Check sheet for the modelled part. Datum: model origin and axes. Units: mm. Coordinates: 2 decimals unless noted, no trailing zeros. Order: outer loops, then holes, each group sorted by start corner. A loop starts at its lowest first (then second) coordinate and runs counter-clockwise, first axis right, second up.
1. Gauge pin test, flat ends, axial feed: pin 1 Ø8 at (y, z) = (-46.5, 55) entering from +X; pin 2 Ø8 at (x, y) = (58, 35.5) entering from -Z; pin 3 Ø6 at (x, z) = (-19.5, 42.5) entering from +Y. Record the tip position at first contact, or that the pin passes through.
2. Cross-section at B-B (x = -5.5). Enter the section's corners in (y, z).
3. Cross-section at D-D (z = 69). Enter the section's corners in (x, y).
4. Cross-section at C-C (y = 25). Enter the section's corners in (x, z), then the cut area to 3 significant figures.
5. Thickness scan on line 1 (X direction, y = 51, z = 74); line 2 (Y direction, x = -110.5, z = 55); line 3 (Y direction, x = 2, z = 70). Record the ranges inside material, lowest first.
6. Cross-section at A-A (z = 39.5). Enter the section's corners in (x, y), then the cut area to 3 significant figures.
```python
from build123d import *

# Parameters (mm, degrees)
F2_DEPTH = 50.8
F4_DEPTH = 254.001


with BuildPart() as f2:
    # F1 (on offset) → F2 (new body)
    with BuildSketch(Plane.XY.offset(25.4)):
        Polygon((0, 127), (-152.4, 0), (0, -76.2), (101.6, 0), align=None)
    extrude(amount=F2_DEPTH)

    # F3 (on face) → F4 (cut, through all)
    with BuildSketch(Plane(origin=(36.576, -48.768, 0), x_dir=(0.8, 0.6, 0), z_dir=(0.6, -0.8, 0))):
        Polygon((-45.72, 25.4), (294.287443, 25.4), (293.713361, 76.2), (-45.72, 50.8), align=None)
    extrude(amount=-F4_DEPTH, mode=Mode.SUBTRACT)


solid = f2.part
```
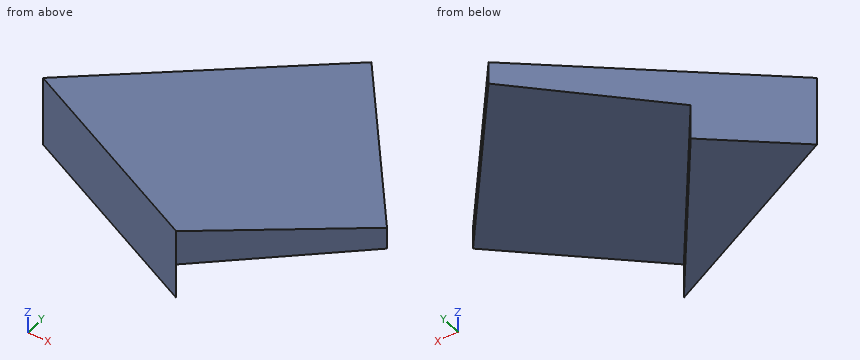
Data:
1. pin 1: stops at x = 44.93
1. pin 2: stops at z = 58.99
1. pin 3: stops at y = -46.2
2. outline: (-73.45, 25.4) - (-68.87, 25.4) - (-68.87, 50.8) - (122.42, 59.39) - (122.42, 76.2) - (-73.45, 76.2) - close
3. outline: (-152.4, 0) - (0, -76.2) - (101.6, 0) - (0, 127) - close
4. outline: (-122.4, 25.4) - (-75.9, 25.4) - (-75.9, 50.8) - (81.6, 60.23) - (81.6, 76.2) - (-122.4, 76.2) - close
4. area: 5,620 mm2
5. line 1: x = -91.2 to 60.8
5. line 2: y = -20.95 to 34.92
5. line 3: y = -74.7 to 124.5
6. outline: (-152.4, 0) - (0, -76.2) - (-93.78, 48.85) - close
6. area: 5,960 mm2
